Read the model definition and answer for the solid it produces. Units are mm, in the model's axes. A direction names the side the tool comes from. Coordinates: 2 decimals unless noted, no trailing zeros. Write each loop counter-clockwise with the first axis right and the second up, starting at its lowest first coordinate (ties: lowest second). Pieces come first, ordered by that corner, then holes. Notation, with made-up numbers: (84.5, -14.75) - (90.5, -14.75) arc R20 cw to (90.5, -2.75) - close; hole circle Ø9 at (11, -21.5). An arc over 180 degrees is marked (long way). Use a Markdown table: item, result.
from build123d import *

# Parameters (mm, degrees)
EXTRUDE_1_DEPTH   = 2
HOLE_WIZARD_M51_D = 5.5
CHAMFER_1_SIZE    = 2


with BuildPart() as part:
    # Эскиз1 → Бобышка-Вытянуть1 (new body)
    with BuildSketch(Plane(origin=(0, 0, 0), x_dir=(1, 0, 0), z_dir=(0, 0, -1))):
        Polygon((0, 0), (0, 60), (60, 60), (60, 40), (20, 40), (20, 0), align=None)
    extrude(amount=EXTRUDE_1_DEPTH)

    # Отверстие с зазором M51 (through all)
    with Locations(Plane(origin=(0, 0, -2), x_dir=(1, 0, 0), z_dir=(0, 0, -1))):
        with Locations((30, 50), (10, 50), (10, 30), (10, 10), (50, 50)):
            Hole(HOLE_WIZARD_M51_D / 2)

    # Фаска1
    chamfer_1_edges = [part.edges().sort_by_distance(p)[0] for p in [
        (0, 0, -1),
        (0, -60, -1),
        (60, -60, -1),
        (60, -40, -1),
        (20, 0, -1),
    ]]
    chamfer(chamfer_1_edges, length=CHAMFER_1_SIZE)


solid = part.part
(1) A cutting plane is placed at B-B, the plane y = -50. Write down the section's boundary in (x, z), and give its area (3 significant figures).
Report:
| item | result |
|---|---|
| outline | (0, -2) - (7.25, -2) - (7.25, 0) - (0, 0) - close; (12.75, -2) - (27.25, -2) - (27.25, 0) - (12.75, 0) - close; (32.75, -2) - (47.25, -2) - (47.25, 0) - (32.75, 0) - close; (52.75, -2) - (60, -2) - (60, 0) - (52.75, 0) - close |
| area | 87.0 mm² |
(2) A cutting plane is placed at D-D, the plane y = -10. Write down the section's boundary in (x, z), and give its area (3 significant figures).
Report:
| item | result |
|---|---|
| outline | (0, -2) - (7.25, -2) - (7.25, 0) - (0, 0) - close; (12.75, -2) - (20, -2) - (20, 0) - (12.75, 0) - close |
| area | 29.0 mm² |
(3) Straight lines are drawn through the part: L1, parallel to Y at x = 10, z = -0.85; L2, parallel to X at y = -50, z = -1.35; L3, parallel to X at y = -30, z = -0.55. For each, find the intervals that lie inside material, in ascending order.
Report:
| item | result |
|---|---|
| L1 | y = -60 to -52.75, -47.25 to -32.75, -27.25 to -12.75, -7.25 to 0 |
| L2 | x = 0 to 7.25, 12.75 to 27.25, 32.75 to 47.25, 52.75 to 60 |
| L3 | x = 0 to 7.25, 12.75 to 20 |
(4) For faces 1 (the cylindrical face through (32.027, -51.859, -0.986)), 2 (the flat face through (39, -40, -1)), determine the directions among +Z, -Z, +X, -X, +Y, -Y from which every point of the face is accessible in a straight line to the end or side of a thin tool.
Report:
| item | result |
|---|---|
| face 1 | +Z, -Z |
| face 2 | +Z, -Z, +X, +Y |
(5) The mould has two halves that part along X. Classify faces 3 (the cylindrical face through (10.358, -52.727, -0.986)), 4 (the flat face through (17, -37, -2)), 5 (the flat face through (19, -1, -1)): pulls with the +X half, pulls with the -X half, needs draft (parallel to the pull), parting line crosses it, or undercut.
Report:
| item | result |
|---|---|
| face 3 | undercut |
| face 4 | needs draft |
| face 5 | pulls with the +X half |
(6) A cutting plane is placed at A-A, the plane x = 30. Write down the section's boundary in (y, z), and give its area (3 significant figures).
Report:
| item | result |
|---|---|
| outline | (-60, -2) - (-52.75, -2) - (-52.75, 0) - (-60, 0) - close; (-47.25, -2) - (-40, -2) - (-40, 0) - (-47.25, 0) - close |
| area | 29.0 mm² |
(7) This flat-tipped pin is pushed along its axis until it touches: P1, Ø1, axis at x = 46, z = -1, coming from the +Y side. Where does it stop, or does it pass through?
Report:
| item | result |
|---|---|
| P1 | stops at y = -40 |
(8) A cutting plane is placed at C-C, the plane z = -1.1. Write down the section's boundary in (x, y).
Report:
| item | result |
|---|---|
| outline | (0, -58) - (2, -60) - (58, -60) - (60, -58) - (60, -42) - (58, -40) - (20, -40) - (20, -2) - (18, 0) - (2, 0) - (0, -2) - close; hole circle Ø5.5 at (10, -50); hole circle Ø5.5 at (10, -30); hole circle Ø5.5 at (10, -10); hole circle Ø5.5 at (30, -50); hole circle Ø5.5 at (50, -50) |
